Build history of the part. All positions in model axes, mm. Face numbers are marked on the shaded views. A direction names the side the tool comes from. Round coordinates to 2 decimals unless told otherwise and drop trailing zeros. Write each loop counter-clockwise with the first axis right and the second up, starting at its lowest first coordinate (ties: lowest second). Pieces come first, ordered by that corner, then holes.
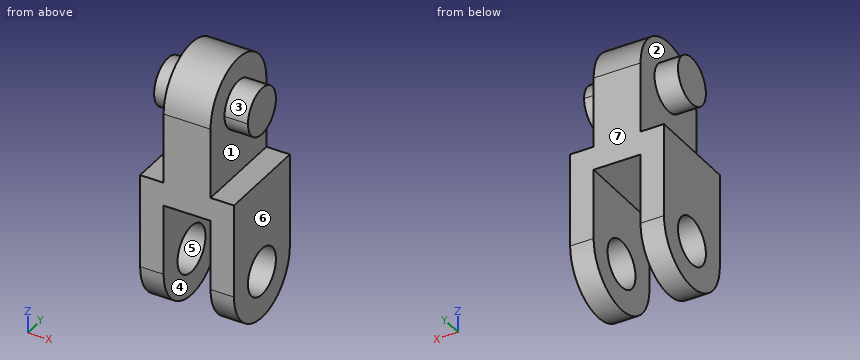
from build123d import *

# Parameters (mm, degrees)
BOSS_EXTRUDE1_DEPTH          = 10
SKETCH2_W                    = 2.5
SKETCH2_H                    = 7.5
CUT_EXTRUDE1_DEPTH           = 31.923292192
SKETCH3_W                    = 5
SKETCH3_H                    = 7.5
CUT_EXTRUDE2_DEPTH           = 31.923292192
SKETCH4_W                    = 2.5
SKETCH4_H                    = 7.5
CUT_EXTRUDE3_DEPTH           = 31.923292192
SKETCH5_W                    = 2.5
SKETCH5_H                    = 2.5
SKETCH6_W                    = 2.5
SKETCH6_H                    = 2.5
F_5_0_5_DIAMETER_HOLE1_D     = 5
F_5_0_5_DIAMETER_HOLE1_DEPTH = 2.5
F_5_0_5_DIAMETER_HOLE2_D     = 5
F_5_0_5_DIAMETER_HOLE2_DEPTH = 2.5
SKETCH11_W                   = 5
SKETCH11_H                   = 5.816268322
CUT_EXTRUDE4_DEPTH           = 10
CUT_EXTRUDE5_DEPTH           = 2.5
CUT_EXTRUDE6_DEPTH           = 2.5


with BuildPart() as part:
    # Sketch1 → Boss-Extrude1 (new body)
    with BuildSketch(Plane(origin=(0, 0, 0), x_dir=(0, -1, 0), z_dir=(-1, 0, 0))):
        with BuildLine():
            Line((0, 22.5), (0, 5))
            ThreePointArc((0, 5), (5, 0), (10, 5))
            Line((10, 5), (10, 22.5))
            ThreePointArc((10, 22.5), (5, 27.5), (0, 22.5))
        make_face()
    extrude(amount=-BOSS_EXTRUDE1_DEPTH)

    # Sketch2 → Cut-Extrude1 (cut, through all)
    with BuildSketch(Plane(origin=(0, 0, 0), x_dir=(-1, 0, 0), z_dir=(0, 1, 0))):
        with Locations((-1.25, 18.75)):
            Rectangle(SKETCH2_W, SKETCH2_H)
    extrude(amount=-CUT_EXTRUDE1_DEPTH, mode=Mode.SUBTRACT)

    # Sketch3 → Cut-Extrude2 (cut, through all)
    with BuildSketch(Plane(origin=(0, 0, 0), x_dir=(-1, 0, 0), z_dir=(0, 1, 0))):
        with Locations((-5, 8.75)):
            Rectangle(SKETCH3_W, SKETCH3_H)
    extrude(amount=-CUT_EXTRUDE2_DEPTH, mode=Mode.SUBTRACT)

    # Sketch4 → Cut-Extrude3 (cut, through all)
    with BuildSketch(Plane(origin=(0, 0, 0), x_dir=(-1, 0, 0), z_dir=(0, 1, 0))):
        with Locations((-8.75, 18.75)):
            Rectangle(SKETCH4_W, SKETCH4_H)
    extrude(amount=-CUT_EXTRUDE3_DEPTH, mode=Mode.SUBTRACT)

    # Sketch5 → Revolve1 (revolve)
    with BuildSketch(Plane.XY.offset(22.5)):
        with Locations((8.75, -3.75)):
            Rectangle(SKETCH5_W, SKETCH5_H)
    revolve(axis=Axis((7.5, -5, 22.5), (1, 0, 0)))

    # Sketch6 → Revolve2 (revolve)
    with BuildSketch(Plane.XY.offset(22.5)):
        with Locations((1.25, -3.75)):
            Rectangle(SKETCH6_W, SKETCH6_H)
    revolve(axis=Axis((0, -5, 22.5), (1, 0, 0)))

    # Ø5.0 (5) Diameter Hole1
    with Locations(Plane.ZY):
        with Locations((5, -5)):
            Hole(F_5_0_5_DIAMETER_HOLE1_D / 2, depth=F_5_0_5_DIAMETER_HOLE1_DEPTH)

    # Ø5.0 (5) Diameter Hole2
    with Locations(Plane(origin=(10, 0, 0), x_dir=(0, 0, -1), z_dir=(1, 0, 0))):
        with Locations((-5, -5)):
            Hole(F_5_0_5_DIAMETER_HOLE2_D / 2, depth=F_5_0_5_DIAMETER_HOLE2_DEPTH)

    # Sketch11 → Cut-Extrude4 (cut)
    with BuildSketch(Plane.XZ.offset(10)):
        with Locations((5, 2.091865839)):
            Rectangle(SKETCH11_W, SKETCH11_H)
    extrude(amount=-CUT_EXTRUDE4_DEPTH, mode=Mode.SUBTRACT)

    # Sketch12 → Cut-Extrude5 (cut)
    with BuildSketch(Plane(origin=(10, 0, 0), x_dir=(0, 0, -1), z_dir=(1, 0, 0))):
        with BuildLine():
            Line((-22.5, -7.5), (-22.5, -10.000084715))
            ThreePointArc((-22.5, -10.000084715), (-27.500042357, -5.000042357), (-22.5, 0))
            Line((-22.5, 0), (-22.5, -2.500084715))
            ThreePointArc((-22.5, -2.500084715), (-24.999957643, -5.000042357), (-22.5, -7.5))
        make_face()
    extrude(amount=-CUT_EXTRUDE5_DEPTH, mode=Mode.SUBTRACT)

    # Sketch13 → Cut-Extrude6 (cut)
    with BuildSketch(Plane.ZY):
        with BuildLine():
            Line((22.5, 0), (22.5, -2.5))
            ThreePointArc((22.5, -2.5), (25, -5), (22.5, -7.5))
            Line((22.5, -7.5), (22.5, -10))
            ThreePointArc((22.5, -10), (27.5, -5), (22.5, 0))
        make_face()
    extrude(amount=-CUT_EXTRUDE6_DEPTH, mode=Mode.SUBTRACT)


solid = part.part
1) Slice it at C-C (z = 5.5). Write the cut outline in (x, y).
Results:
outline: (0, -10) - (2.5, -10) - (2.5, -7.45) - (0, -7.45) - close; (0, -2.55) - (2.5, -2.55) - (2.5, 0) - (0, 0) - close; (7.5, -10) - (10, -10) - (10, -7.45) - (7.5, -7.45) - close; (7.5, -2.55) - (10, -2.55) - (10, 0) - (7.5, 0) - close
2) Which spindle directions (+Z, -Z, +X, -X, +Y, -Y) get a long thin tool onto all of the face, cutting with end or side? Do the marked faces 1, 2, 3 and 4. Say none if no direction does.
Results:
face 1: +X
face 2: -X
face 3: +Z, +X
face 4: -Z, +Y, -Y
3) Mould opens along Y. For the marked faces 5, 6 and 7 say: released by +Y, released by -Y, zero draft, split by the parting line, or undercut.
Results:
face 5: undercut
face 6: zero draft
face 7: released by +Y
4) Slice it at A-A (x = 9). Count the separate pieces of the cut face and the enclosed holes in it, plus the area to 3 significant figures.
Results:
separate pieces: 2
enclosed holes: 1
area: 139 mm2
5) Wall check: L1, parallel to Z at x = 9.15, y = -5; L2, parallel to Y at x = 0.8, z = 5; L3, parallel to Z at x = 9.5, y = -4. Give the ranges that are in metal, low to high.
Results:
L1: z = 0 to 2.5, 7.5 to 15, 20 to 25
L2: y = -10 to -7.5, -2.5 to 0
L3: z = 0.1 to 2.71, 7.29 to 15, 20.21 to 24.79
6) Slice it at B-B (y = -5). Write the cut outline in (x, z), plus the area to 3 significant figures.
Results:
outline: (0, 0) - (2.5, 0) - (2.5, 2.5) - (0, 2.5) - close; (0, 7.5) - (2.5, 7.5) - (2.5, 12.5) - (7.5, 12.5) - (7.5, 7.5) - (10, 7.5) - (10, 15) - (7.5, 15) - (7.5, 20) - (10, 20) - (10, 25) - (7.5, 25) - (7.5, 27.5) - (2.5, 27.5) - (2.5, 25) - (0, 25) - (0, 20) - (2.5, 20) - (2.5, 15) - (0, 15) - close; (7.5, 0) - (10, 0) - (10, 2.5) - (7.5, 2.5) - close
area: 150 mm2
7) Pin check, flat tips, straight feed: pin 1 Ø0.8 at (x, y) = (1, -6) entering from +Z; pin 2 Ø2 at (x, y) = (4.5, -8.5) entering from -Z; pin 3 Ø1.2 at (x, y) = (8, -3.5) entering from +Z. Stop position of each tip, or through.
Results:
pin 1: stops at z = 24.93
pin 2: stops at z = 12.5
pin 3: stops at z = 27.36
8) Slice it at D-D (z = 21.25). Write the cut outline in (x, y).
Results:
outline: (0, -7.17) - (2.5, -7.17) - (2.5, -10) - (7.5, -10) - (7.5, -7.17) - (10, -7.17) - (10, -2.83) - (7.5, -2.83) - (7.5, 0) - (2.5, 0) - (2.5, -2.83) - (0, -2.83) - close
